Source: CAD feature listing. Evaluate the final solid. Frame: model axes, mm. Coordinates: 2 decimals unless noted, no trailing zeros. Order: outer loops, then holes, each group sorted by start corner. A loop starts at its lowest first (then second) coordinate and runs counter-clockwise, first axis right, second up. Notation, with made-up numbers: (-17.75, 75) -> (1.25, 75) arc R9 ccw to (1.25, 90) -> close; hole circle Ø10 at (70, -39). An arc over 180 degrees is marked (long way). Put each result on its own line as item: value.
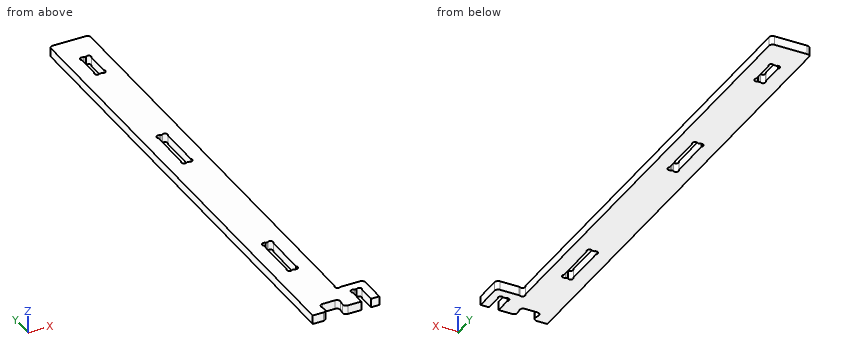
from build123d import *

# Parameters (mm, degrees)
BOSS_EXTRUDE1_DEPTH = 18
CUT_EXTRUDE1_DEPTH  = 19
CUT_EXTRUDE2_DEPTH  = 19
CUT_EXTRUDE3_DEPTH  = 19
LPATTERN1_COUNT     = 2
LPATTERN1_PITCH     = 400
FILLET1_R           = 7


with BuildPart() as part:
    # Sketch1 → Boss-Extrude1 (new body)
    with BuildSketch(Plane.XY):
        with BuildLine():
            Line((0, 0), (29.493640444, 0))
            Line((29.493640444, 0), (25.413640444, 25.5))
            Line((25.413640444, 25.5), (66.586359556, 25.5))
            Line((66.586359556, 25.5), (62.506359556, 0))
            Line((62.506359556, 0), (134, 0))
            Line((134, 0), (134, 60))
            Line((134, 60), (88.745587739, 60))
            ThreePointArc((88.745587739, 60), (87.392597488, 59.813462099), (86.140560822, 59.267766953))
            ThreePointArc((86.140560822, 59.267766953), (80, 60), (79.267766953, 66.140560822))
            ThreePointArc((79.267766953, 66.140560822), (79.813462099, 67.392597488), (80, 68.745587739))
            Line((80, 68.745587739), (80, 1000))
            Line((80, 1000), (0, 1000))
            Line((0, 1000), (0, 0))
        make_face()
    extrude(amount=BOSS_EXTRUDE1_DEPTH)

    # Sketch2 → Cut-Extrude1 (cut, through all)
    with BuildSketch(Plane.XY):
        with BuildLine():
            Line((30.5, 642.748771852), (30.5, 557.251228148))
            ThreePointArc((30.5, 557.251228148), (30.400327171, 556.660561143), (30.11234721, 556.135309084))
            ThreePointArc((30.11234721, 556.135309084), (30.5, 549.5), (37.135309084, 549.11234721))
            ThreePointArc((37.135309084, 549.11234721), (37.660561143, 549.400327171), (38.251228148, 549.5))
            Line((38.251228148, 549.5), (41.748771852, 549.5))
            ThreePointArc((41.748771852, 549.5), (42.339438857, 549.400327171), (42.864690916, 549.11234721))
            ThreePointArc((42.864690916, 549.11234721), (49.5, 549.5), (49.88765279, 556.135309084))
            ThreePointArc((49.88765279, 556.135309084), (49.599672829, 556.660561143), (49.5, 557.251228148))
            Line((49.5, 557.251228148), (49.5, 642.748771852))
            ThreePointArc((49.5, 642.748771852), (49.599672829, 643.339438857), (49.88765279, 643.864690916))
            ThreePointArc((49.88765279, 643.864690916), (49.5, 650.5), (42.864690916, 650.88765279))
            ThreePointArc((42.864690916, 650.88765279), (42.339438857, 650.599672829), (41.748771852, 650.5))
            Line((41.748771852, 650.5), (38.251228148, 650.5))
            ThreePointArc((38.251228148, 650.5), (37.660561143, 650.599672829), (37.135309084, 650.88765279))
            ThreePointArc((37.135309084, 650.88765279), (30.5, 650.5), (30.11234721, 643.864690916))
            ThreePointArc((30.11234721, 643.864690916), (30.400327171, 643.339438857), (30.5, 642.748771852))
        make_face()
    cut_extrude1 = extrude(amount=CUT_EXTRUDE1_DEPTH, mode=Mode.SUBTRACT)

    # Sketch3 → Cut-Extrude2 (cut, through all)
    with BuildSketch(Plane.XY):
        with BuildLine():
            Line((98, 0), (117, 0))
            Line((117, 0), (117, 32.748771852))
            ThreePointArc((117, 32.748771852), (117.099672829, 33.339438857), (117.38765279, 33.864690916))
            ThreePointArc((117.38765279, 33.864690916), (117, 40.5), (110.364690916, 40.88765279))
            ThreePointArc((110.364690916, 40.88765279), (109.839438857, 40.599672829), (109.248771852, 40.5))
            Line((109.248771852, 40.5), (105.751228148, 40.5))
            ThreePointArc((105.751228148, 40.5), (105.160561143, 40.599672829), (104.635309084, 40.88765279))
            ThreePointArc((104.635309084, 40.88765279), (98, 40.5), (97.61234721, 33.864690916))
            ThreePointArc((97.61234721, 33.864690916), (97.900327171, 33.339438857), (98, 32.748771852))
            Line((98, 32.748771852), (98, 0))
        make_face()
    extrude(amount=CUT_EXTRUDE2_DEPTH, mode=Mode.SUBTRACT)

    # Sketch4 → Cut-Extrude3 (cut, through all)
    with BuildSketch(Plane.XY):
        with BuildLine():
            Line((30.5, 932.748771852), (30.5, 887.251228148))
            ThreePointArc((30.5, 887.251228148), (30.400327171, 886.660561143), (30.11234721, 886.135309084))
            ThreePointArc((30.11234721, 886.135309084), (30.5, 879.5), (37.135309084, 879.11234721))
            ThreePointArc((37.135309084, 879.11234721), (37.660561143, 879.400327171), (38.251228148, 879.5))
            Line((38.251228148, 879.5), (41.748771852, 879.5))
            ThreePointArc((41.748771852, 879.5), (42.339438857, 879.400327171), (42.864690916, 879.11234721))
            ThreePointArc((42.864690916, 879.11234721), (49.5, 879.5), (49.88765279, 886.135309084))
            ThreePointArc((49.88765279, 886.135309084), (49.599672829, 886.660561143), (49.5, 887.251228148))
            Line((49.5, 887.251228148), (49.5, 932.748771852))
            ThreePointArc((49.5, 932.748771852), (49.599672829, 933.339438857), (49.88765279, 933.864690916))
            ThreePointArc((49.88765279, 933.864690916), (49.5, 940.5), (42.864690916, 940.88765279))
            ThreePointArc((42.864690916, 940.88765279), (42.339438857, 940.599672829), (41.748771852, 940.5))
            Line((41.748771852, 940.5), (38.251228148, 940.5))
            ThreePointArc((38.251228148, 940.5), (37.660561143, 940.599672829), (37.135309084, 940.88765279))
            ThreePointArc((37.135309084, 940.88765279), (30.5, 940.5), (30.11234721, 933.864690916))
            ThreePointArc((30.11234721, 933.864690916), (30.400327171, 933.339438857), (30.5, 932.748771852))
        make_face()
    extrude(amount=CUT_EXTRUDE3_DEPTH, mode=Mode.SUBTRACT)

    # LPattern1: Cut-Extrude1 ×2
    with Locations(*[(0, -i * LPATTERN1_PITCH, 0) for i in range(1, LPATTERN1_COUNT)]):
        add(cut_extrude1, mode=Mode.SUBTRACT)

    # Fillet1
    fillet1_edges = [part.edges().sort_by_distance(p)[0] for p in [
        (29.493640444, 0, 9),
        (25.413640444, 25.5, 9),
        (66.586359556, 25.5, 9),
        (62.506359556, 0, 9),
        (134, 60, 9),
        (80, 1000, 9),
        (0, 1000, 9),
    ]]
    fillet(fillet1_edges, radius=FILLET1_R)


solid = part.part
1. First-contact query: pin 1 (5.5 mm diameter, centred on x = 103.5, z = 8, fed in from +Y); pin 2 (5.5 mm diameter, centred on y = 583.5, z = 12, fed in from +X); pin 3 (3 mm diameter, centred on x = 39.5, z = 4.5, fed in from -Y). Flat tips, straight axial feed; report the tip coordinate or a pass-through.
Numbers:
pin 1: stops at y = 60
pin 2: stops at x = 80
pin 3: stops at y = 25.5
2. Cut plane A-A on z = 4.25. Count the separate pieces of the cut face and the enclosed holes in it, plus the area to 3 significant figures.
Numbers:
separate pieces: 1
enclosed holes: 3
area: 76,300 mm2
3. Cut plane B-B on y = 665. Output: boundary loops of the cut face in (x, z), plus the area to 3 significant figures.
Numbers:
outline: (0, 0) -> (80, 0) -> (80, 18) -> (0, 18) -> close
area: 1,440 mm2
4. Ray query, line 1 along Y through (x, z) = (46, 9.5); line 2 along X through (y, z) = (613, 14.25); line 3 along Y through (x, z) = (34.5, 14.5). Return the intervals inside material, ascending.
Numbers:
line 1: y = 25.5 to 148.04, 251.96 to 548.04, 651.96 to 878.04, 941.96 to 1000
line 2: x = 0 to 30.5, 49.5 to 80
line 3: y = 25.5 to 148.06, 251.94 to 548.06, 651.94 to 878.06, 941.94 to 1000
